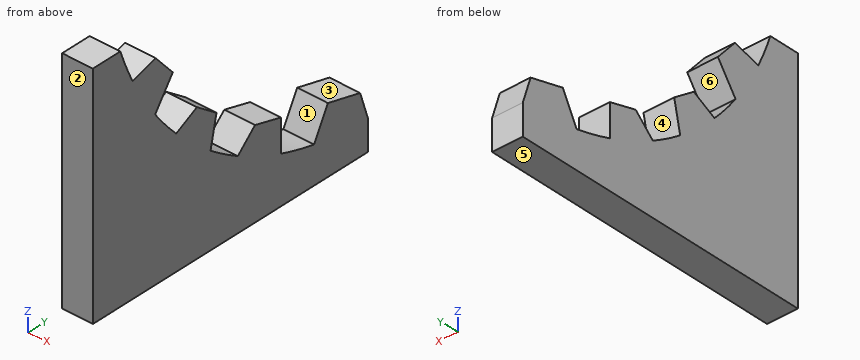
from build123d import *

# Parameters (mm, degrees)
F1_DEPTH = 25


with BuildPart() as f1:
    # F0 (on Right) → F1 (new body)
    with BuildSketch(Plane.YZ):
        with BuildLine():
            Line((-36.035504, 106.236686), (-36.035504, -80.763314))
            Line((-36.035504, -80.763314), (213.964496, -80.763314))
            Line((213.964496, -80.763314), (213.964496, -55.763314))
            Line((213.964496, -55.763314), (206.940986, -33.974228))
            Line((206.940986, -33.974228), (177.683763, -26.659922))
            Line((177.683763, -26.659922), (165.041714, -50.65876))
            ThreePointArc((165.041714, -50.65876), (149.817431, -46.919692), (134.873256, -42.183545))
            Line((134.873256, -42.183545), (134.873256, -15.630545))
            Line((134.873256, -15.630545), (111.362994, -9.36128))
            Line((111.362994, -9.36128), (95.788479, -24.225105))
            ThreePointArc((95.788479, -24.225105), (83.106224, -16.399421), (70.940202, -7.793098))
            Line((70.940202, -7.793098), (76.35881, 17.283693))
            Line((76.35881, 17.283693), (58.595493, 30.344954))
            Line((58.595493, 30.344954), (39.715554, 20.487944))
            ThreePointArc((39.715554, 20.487944), (29.767414, 31.970469), (20.574449, 44.066057))
            Line((20.574449, 44.066057), (36.652576, 66.916481))
            Line((36.652576, 66.916481), (20.979062, 85.202247))
            Line((20.979062, 85.202247), (0, 78.992389))
            ThreePointArc((0, 78.992389), (-5.940015, 92.443497), (-11.035504, 106.236686))
            Line((-11.035504, 106.236686), (-36.035504, 106.236686))
        make_face()
    extrude(amount=F1_DEPTH)


solid = f1.part
Model file for the job. Use its own axes, mm. Face numbers are marked on the shaded views. A direction names the side the tool comes from. Give positions to 0.01 mm unless a question says otherwise; leave off trailing zeros. Loops run counter-clockwise (first coordinate to the right, second up) from the corner with the lowest first, then second, coordinate; pieces in that order, holes last. Notation, with made-up numbers: (66, 75.25) -> (105, 75.25) arc R23 ccw to (105, 86.25) -> close; hole circle Ø11 at (24, 23). An arc over 180 degrees is marked (long way). Use a Markdown table: item, result. Add a question column.
(1) Slice it at A-A on x = 4.25. List the corners of the cut face in (y, z).
(2) Wall check: line 1 along Y through (x, z) = (6.75, -19.5); line 2 along Y through (x, z) = (7.25, 23); line 3 along Y through (x, z) = (18, -7). Give the ranges that are in metal, low to high.
(3) Mould opens along Z. For the marked faces 3, 4, 5 and 6 say: +Z half, -Z half, draft (parallel to the pull), parting line (faces both ways), or undercut.
(4) Slice it at B-B on y = 187. List the corners of the cut face in (x, z), and give its area (3 significant figures).
(5) Tool access for the marked faces 1 and 2: list every direction of +Z, -Z, +X, -X, +Y, -Y with a clear straight run to the whole face (end or side of a thin tool).
(6) Drop flat-ended pins along their axis: pin 1 Ø10 at (x, z) = (9.5, -0.5) entering from +Y; pin 2 Ø3 at (x, z) = (4.5, 17) entering from +Y. Give the stop position or say it passes through.
(7) Slice it at C-C on z = -4. List the corners of the cut face in (x, y), and give its area (3 significant figures).
Filled sheet:
| question | item | result |
|---|---|---|
| 1 | outline | (-36.04, -80.76) -> (213.96, -80.76) -> (213.96, -55.76) -> (206.94, -33.97) -> (177.68, -26.66) -> (165.04, -50.66) arc R237.29 cw to (134.87, -42.18) -> (134.87, -15.63) -> (111.36, -9.36) -> (95.79, -24.23) arc R237.29 cw to (70.94, -7.79) -> (76.36, 17.28) -> (58.6, 30.34) -> (39.72, 20.49) arc R237.29 cw to (20.57, 44.07) -> (36.65, 66.92) -> (20.98, 85.2) -> (0, 78.99) arc R237.29 cw to (-11.04, 106.24) -> (-36.04, 106.24) -> close |
| 2 | line 1 | -36.04 to 87.92, 100.74 to 134.87 |
| 2 | line 2 | -36.04 to 37.43, 44.53 to 68.58 |
| 2 | line 3 | -36.04 to 71.11 |
| 3 | face 3 | +Z half |
| 3 | face 4 | undercut |
| 3 | face 5 | -Z half |
| 3 | face 6 | undercut |
| 4 | outline | (0, -80.76) -> (25, -80.76) -> (25, -28.99) -> (0, -28.99) -> close |
| 4 | area | 1,290 mm2 |
| 5 | face 1 | +Z, +X, -X |
| 5 | face 2 | +Z, -Z, +X, -X, -Y |
| 6 | pin 1 | y = 73.6 |
| 6 | pin 2 | y = 76.36 |
| 7 | outline | (0, -36.04) -> (25, -36.04) -> (25, 71.76) -> (0, 71.76) -> close |
| 7 | area | 2,690 mm2 |
